```python
from build123d import *

# Parameters (mm, degrees)
SKETCH1_R                = 47.5
BOSS_EXTRUDE1_DEPTH      = 5
FILLET1_R                = 2
BOSS_EXTRUDE2_DEPTH      = 60
BOSS_EXTRUDE2_DEPTH_BACK = 50
SKETCH2_R                = 7.5


with BuildPart() as part:
    # Sketch1 → Boss-Extrude1 (new body)
    with BuildSketch(Plane(origin=(0, 0, 0), x_dir=(0, 0, -1), z_dir=(1, 0, 0))):
        Circle(SKETCH1_R)
    extrude(amount=BOSS_EXTRUDE1_DEPTH)

    # Fillet1
    fillet1_edges = [part.edges().sort_by_distance(p)[0] for p in [
        (0, 0, 47.5),
        (5, 0, 47.5),
    ]]
    fillet(fillet1_edges, radius=FILLET1_R)

    # Sketch2 → Boss-Extrude2 (add, two sides: drawn at the far end of the back side and taken through both)
    with BuildSketch(Plane.XY.offset(-BOSS_EXTRUDE2_DEPTH_BACK)):
        with Locations((12, 0)):
            Circle(SKETCH2_R)
    extrude(amount=BOSS_EXTRUDE2_DEPTH + BOSS_EXTRUDE2_DEPTH_BACK)


solid = part.part
```
Source: CAD feature listing. Evaluate the final solid. Frame: model axes, mm. Give positions to 0.01 mm unless a question says otherwise; leave off trailing zeros. Order: outer loops, then holes, each group sorted by start corner. A loop starts at its lowest first (then second) coordinate and runs counter-clockwise, first axis right, second up.
(1) Contact query for flat-ended pins moving along their axis: P1, Ø1, axis at y = 24, z = 34, coming from the -X side; P2, Ø1.5, axis at y = 28, z = 18, coming from the +X side; P3, Ø2, axis at x = 2.5, y = -2, coming from the +Z side; P4, Ø1, axis at x = 4.5, y = -4.5, coming from the -Z side. Output: stop coordinate, or through.
(2) Section query B-B (x = 12). Return the cut outline in (y, z).
(3) Section query C-C (y = 0). Return the cut outline in (x, z).
(4) Section query A-A (z = 0). Return the cut outline in (x, y).
(5) Material intervals for line 1 along X through (y, z) = (-9.5, -12); line 2 along Y through (x, z) = (12.5, 41); line 3 along X through (y, z) = (1, -16), sorted ascending.
(6) Pull-direction query (X, two-part tool) for faces 1 (the face through (12, 0, 60)), 2 (the face through (0, 1, 1)), 3 (the face through (18.93, -2.87, 4.23)); classes: +X half, -X half, draft (parallel to the pull), parting line (faces both ways), or undercut.
Outcome:
1. P1: stops at x = 0
1. P2: stops at x = 5
1. P3: stops at z = 47.49
1. P4: stops at z = -47.02
2. outline: (-7.5, -50) - (7.5, -50) - (7.5, 60) - (-7.5, 60) - close
3. outline: (0, -45.5) arc R2 ccw to (2, -47.5) - (3, -47.5) arc R2 ccw to (4.5, -46.82) - (4.5, -50) - (19.5, -50) - (19.5, 60) - (4.5, 60) - (4.5, 46.82) arc R2 ccw to (3, 47.5) - (2, 47.5) arc R2 ccw to (0, 45.5) - close
4. outline: (0, -45.5) arc R2 ccw to (2, -47.5) - (3, -47.5) arc R2 ccw to (5, -45.5) - (5, -2.69) arc R7.5 ccw (long way) to (5, 2.69) - (5, 45.5) arc R2 ccw to (3, 47.5) - (2, 47.5) arc R2 ccw to (0, 45.5) - close
5. line 1: x = 0 to 5
5. line 2: y = -7.48 to 7.48
5. line 3: x = 0 to 19.43
6. face 1: draft
6. face 2: -X half
6. face 3: undercut
